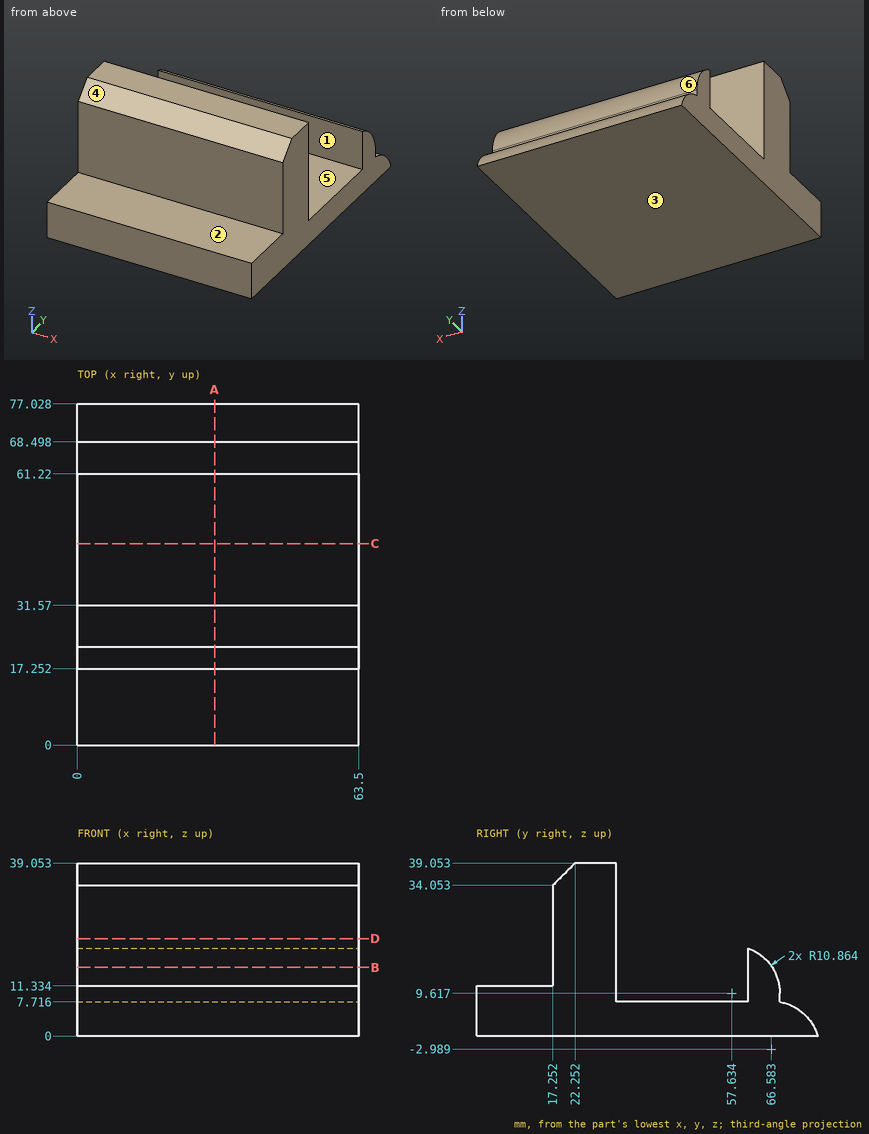
For this review, use the dimensioned drawing (mm, ordinates from the lowest corner) and the shaded views. A direction names the side the tool comes from. Round coordinates to 2 decimals unless told otherwise and drop trailing zeros. Write each loop counter-clockwise with the first axis right and the second up, starting at its lowest first coordinate (ties: lowest second). Pieces come first, ordered by that corner, then holes. Notation, with made-up numbers: (14.25, -33.75) -> (53.25, -33.75) arc R17 ccw to (53.25, -5.75) -> close; hole circle Ø6 at (39.25, 29). An arc over 180 degrees is marked (long way). Use CSV: the item, a comma, the result in double quotes.
(1) Draft analysis for pull direction Y (two halves, no side actions). For the marked faces 4, 5 and 6, state which applies: +Y half, -Y half, draft (parallel to the pull), parting line (faces both ways), or undercut.
Computed values:
face 4,"-Y half"
face 5,"undercut"
face 6,"+Y half"
(2) Consider section A-A, the plane x = 31. Give the boundary of the cut face in (y, z) (1 decimal).
Computed values:
outline,"(0, 0) -> (77, 0) arc R10.9 ccw to (68.5, 7.7) -> (68.5, 9.6) arc R10.9 ccw to (61.2, 19.9) -> (61.2, 7.7) -> (31.6, 7.7) -> (31.6, 39.1) -> (22.3, 39.1) -> (17.3, 34.1) -> (17.3, 11.3) -> (0, 11.3) -> close"
(3) Consider section B-B, the plane z = 15.5. Give the boundary of the cut face in (x, y), plus the area to 3 significant figures.
Computed values:
outline,"(0, 17.25) -> (63.5, 17.25) -> (63.5, 31.57) -> (0, 31.57) -> close; (0, 61.22) -> (63.5, 61.22) -> (63.5, 66.77) -> (0, 66.77) -> close"
area,"1,260 mm²"
(4) To check wall thickness, follow L1, parallel to Y at x = 36.5, z = 8; L2, parallel to Z at x = 56, y = 58.5 (1 decimal); L3, parallel to Z at x = 20, y = 8. State the ranges of each line that lie inside material, in increasing order. Write a range as [from, to].
Computed values:
L1,"[0, 31.57], [61.22, 68.5]"
L2,"[0, 7.7]"
L3,"[0, 11.33]"
(5) Clearance check with flat-ended pins moving along their axes: P1, Ø11.5, axis at x = 19.5, z = 27.5, coming from the -Y side; P2, Ø19, axis at x = 18.5, y = 12.5, coming from the +Z side; P3, Ø9.5, axis at x = 17, z = 15, coming from the -Y side; P4, Ø9.5, axis at x = 22, z = 21.5, coming from the +Y side. State where each tip first meets the part, or that it passes through.
Computed values:
P1,"y = 17.25"
P2,"z = 38.8"
P3,"y = 0"
P4,"y = 65.83"
(6) For the marked faces 1, 2 and 3, list the 3-axis set-ups (+Z, -Z, +X, -X, +Y, -Y) from which the entire face can be reached by the end or side of a thin tool; tool diameter is ignored.
Computed values:
face 1,"+Z, +X, -X"
face 2,"+Z, +X, -X, -Y"
face 3,"-Z, +X, -X, +Y, -Y"
(7) Consider section C-C, the plane y = 45.5. Give the boundary of the cut face in (x, z) (1 decimal).
Computed values:
outline,"(0, 0) -> (63.5, 0) -> (63.5, 7.7) -> (0, 7.7) -> close"
(8) Consider section D-D, the plane z = 22. Give the boundary of the cut face in (x, y), plus the area to 3 significant figures.
Computed values:
outline,"(0, 17.25) -> (63.5, 17.25) -> (63.5, 31.57) -> (0, 31.57) -> close"
area,"909 mm²"
